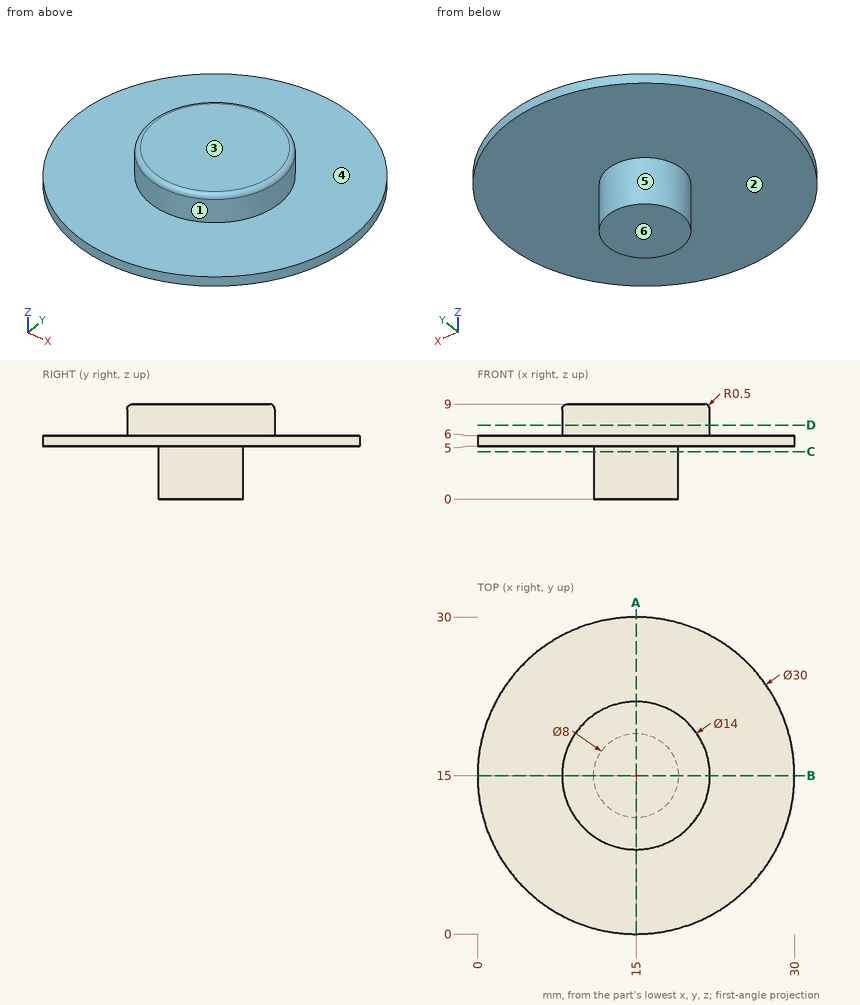
Could you check a few things on this drawing? It's one solid part, dimensions in mm from its lowest x, y, z. A direction names the side the tool comes from. Round coordinates to 2 decimals unless told otherwise and drop trailing zeros. Order: outer loops, then holes, each group sorted by start corner. A loop starts at its lowest first (then second) coordinate and runs counter-clockwise, first axis right, second up.
(1) Please list where these lines run through material, in increasing order: line 1 along Z through (x, y) = (6.75, 20.5); line 2 along Z through (x, y) = (15.25, 20.5); line 3 along X through (y, z) = (4.5, 5.75).
Response values:
line 1: z = 5 to 6
line 2: z = 5 to 9
line 3: x = 4.29 to 25.71
(2) Imagine slicing it at C-C (z = 4.5). Write out the boundary of the cut face in (x, y), plus the area to 3 significant figures.
Response values:
outline: circle Ø8 at (15, 15)
area: 50.3 mm2
(3) Imagine slicing it at D-D (z = 7). Write out the boundary of the cut face in (x, y), plus the area to 3 significant figures.
Response values:
outline: circle Ø14 at (15, 15)
area: 154 mm2
(4) Which directions (+Z, -Z, +X, -X, +Y, -Y) give clear straight access to the entire face, cutting with the end or side of a thin tool? Please do the marked faces 4, 5 and 6.
Response values:
face 4: +Z
face 5: -Z
face 6: -Z, +X, -X, +Y, -Y
(5) Imagine slicing it at A-A (x = 15). Write out the boundary of the cut face in (y, z), plus the area to 3 significant figures.
Response values:
outline: (0, 5) - (11, 5) - (11, 0) - (19, 0) - (19, 5) - (30, 5) - (30, 6) - (22, 6) - (22, 8.5) arc R0.5 ccw to (21.5, 9) - (8.5, 9) arc R0.5 ccw to (8, 8.5) - (8, 6) - (0, 6) - close
area: 112 mm2
(6) I'm going to push flat-ended pins straight in: pin 1 (2 mm diameter, centred on y = 14, z = 2, fed in from +X); pin 2 (10 mm diameter, centred on x = 13, y = 16.5, fed in from -Z); pin 3 (10 mm diameter, centred on x = 25, y = 10.5, fed in from -Z). Where does each tip first touch, or does it pass through?
Response values:
pin 1: stops at x = 19
pin 2: stops at z = 0
pin 3: stops at z = 5
(7) If we mould it in two halves opening along Z, with no side actions, what happens to the marked faces 1, 2 and 3? For each: released by +Z, released by -Z, zero draft, split by the parting line, or undercut.
Response values:
face 1: zero draft
face 2: released by -Z
face 3: released by +Z
